```python
from build123d import *

# Parameters (mm, degrees)
SKETCH1_W           = 16
SKETCH1_H           = 46
BOSS_EXTRUDE1_DEPTH = 1.6
SKETCH3_W           = 10
SKETCH3_H           = 26
CUT_EXTRUDE2_DEPTH  = 1.6
CHAMFER2_SIZE       = 2
SKETCH4_R           = 1.5
CUT_EXTRUDE3_DEPTH  = 1.6


with BuildPart() as part:
    # Sketch1 → Boss-Extrude1 (new body)
    with BuildSketch(Plane(origin=(0, 0, 0), x_dir=(1, 0, 0), z_dir=(0, 1, 0))):
        Rectangle(SKETCH1_W, SKETCH1_H)
    extrude(amount=BOSS_EXTRUDE1_DEPTH)

    # Sketch3 → Cut-Extrude2 (cut)
    with BuildSketch(Plane(origin=(0, 1.6, 0), x_dir=(1, 0, 0), z_dir=(0, 1, 0))):
        with Locations((0, 6)):
            Rectangle(SKETCH3_W, SKETCH3_H)
    extrude(amount=-CUT_EXTRUDE2_DEPTH, mode=Mode.SUBTRACT)

    # Chamfer2
    chamfer2_edges = [part.edges().sort_by_distance(p)[0] for p in [
        (5, 0.8, 7),
        (5, 0.8, -19),
        (-5, 0.8, -19),
        (-5, 0.8, 7),
    ]]
    chamfer(chamfer2_edges, length=CHAMFER2_SIZE)

    # Sketch4 → Cut-Extrude3 (cut)
    with BuildSketch(Plane(origin=(0, 1.6, 0), x_dir=(1, 0, 0), z_dir=(0, 1, 0))):
        with Locations(Location((0, -10.5, 0), (0, 0, 270))):
            Circle(SKETCH4_R)
    extrude(amount=-CUT_EXTRUDE3_DEPTH, mode=Mode.SUBTRACT)


solid = part.part
```
Geometry: final body of the model. Coordinates: model frame, mm. A direction names the side the tool comes from. Round coordinates to 2 decimals unless told otherwise and drop trailing zeros. Loops run counter-clockwise (first coordinate to the right, second up) from the corner with the lowest first, then second, coordinate; pieces in that order, holes last. Notation, with made-up numbers: (-16.75, -20.75) -> (-3.75, -20.75) arc R19 ccw to (-3.75, 5.25) -> close; hole circle Ø6 at (84.25, -32). An arc over 180 degrees is marked (long way). Use one line per item in the form item = value. Start each with the question number.
1) Section C-C on x = 0. Output: boundary loops of the cut face in (y, z).
2) Section A-A on x = -2.25. Output: boundary loops of the cut face in (y, z), then the cut area to 3 significant figures.
3) Draft query along Z for faces 1 (the flat face through (0, 1, -19)), 2 (the flat face through (-5.4, 0, -0.3)), 3 (the flat face through (0, 1, -23)), 4 (the cylindrical face through (0, 1, 9)). Return one class per face: released by +Z, released by -Z, zero draft, split by the parting line, or undercut.
4) Line query: L1, parallel to X at y = 0.65, z = -5; L2, parallel to X at y = 0.9, z = 10.5; L3, parallel to Z at x = 2.25, y = 1.2. Output: solid intervals per line, ascending.
5) Section D-D on y = 1. Output: boundary loops of the cut face in (x, z).
6) Access query for faces 5 (the flat face through (-4, 1, 6)), 6 (the flat face through (8, 1, 0)). Directions: +Z, -Z, +X, -X, +Y, -Y. A direction counts if a zero-diameter tool reaches every point of the face in a straight line with its end or side. Return the directions, or none.
7) Section B-B on z = 10.5. Output: boundary loops of the cut face in (x, y), then the cut area to 3 significant figures.
Response:
q1.outline = (0, -23) -> (1.6, -23) -> (1.6, -19) -> (0, -19) -> close; (0, 7) -> (1.6, 7) -> (1.6, 9) -> (0, 9) -> close; (0, 12) -> (1.6, 12) -> (1.6, 23) -> (0, 23) -> close
q2.outline = (0, -23) -> (1.6, -23) -> (1.6, -19) -> (0, -19) -> close; (0, 7) -> (1.6, 7) -> (1.6, 23) -> (0, 23) -> close
q2.area = 32.0 mm^2
q3.face_1 = undercut
q3.face_2 = zero draft
q3.face_3 = released by -Z
q3.face_4 = undercut
q4.L1 = -8 to -5, 5 to 8
q4.L2 = -8 to -1.5, 1.5 to 8
q4.L3 = -23 to -19, 7 to 23
q5.outline = (-8, -23) -> (8, -23) -> (8, 23) -> (-8, 23) -> close; hole (-5, -17) -> (-3, -19) -> (3, -19) -> (5, -17) -> (5, 5) -> (3, 7) -> (-3, 7) -> (-5, 5) -> close; hole circle Ø3 at (0, 10.5)
q6.face_5 = +Y, -Y
q6.face_6 = +Z, -Z, +X, +Y, -Y
q7.outline = (-8, 0) -> (-1.5, 0) -> (-1.5, 1.6) -> (-8, 1.6) -> close; (1.5, 0) -> (8, 0) -> (8, 1.6) -> (1.5, 1.6) -> close
q7.area = 20.8 mm^2
